```python
from build123d import *

# Parameters (mm, degrees)
BOX006_W     = 90
BOX006_H     = 90
BOX006_DEPTH = 10
FILLET008_R  = 5
BOX007_W     = 100
BOX007_H     = 100
BOX007_DEPTH = 10
FILLET007_R  = 7
BOX008_W     = 94
BOX008_H     = 94
BOX008_DEPTH = 2
FILLET006_R  = 7


with BuildPart() as fillet008:
    # Box006 → Box006 (new body)
    with BuildSketch(Plane(origin=(5, 5, 3), x_dir=(1, 0, 0), z_dir=(0, 0, 1))):
        with Locations((45, 45)):
            Rectangle(BOX006_W, BOX006_H)
    extrude(amount=BOX006_DEPTH)

    # Fillet008
    fillet008_edges = [fillet008.edges().sort_by_distance(p)[0] for p in [
        (5, 5, 8),
        (5, 95, 8),
        (95, 5, 8),
        (95, 95, 8),
    ]]
    fillet(fillet008_edges, radius=FILLET008_R)


with BuildPart() as body_with_fillets003:
    # Box007 → Box007 (new body)
    with BuildSketch(Plane.XY):
        with Locations((50, 50)):
            Rectangle(BOX007_W, BOX007_H)
    extrude(amount=BOX007_DEPTH)

    # Fillet007
    fillet007_edges = [body_with_fillets003.edges().sort_by_distance(p)[0] for p in [
        (0, 0, 5),
        (0, 100, 5),
        (100, 0, 5),
        (100, 100, 5),
    ]]
    fillet(fillet007_edges, radius=FILLET007_R)


with BuildPart() as wet_palette:
    # Box008 → Box008 (new body)
    with BuildSketch(Plane(origin=(3, 3, 10), x_dir=(1, 0, 0), z_dir=(0, 0, 1))):
        with Locations((47, 47)):
            Rectangle(BOX008_W, BOX008_H)
    extrude(amount=BOX008_DEPTH)

    # Fillet006
    fillet006_edges = [wet_palette.edges().sort_by_distance(p)[0] for p in [
        (3, 3, 11),
        (3, 97, 11),
        (97, 3, 11),
        (97, 97, 11),
    ]]
    fillet(fillet006_edges, radius=FILLET006_R)

    # Fusion003: union Body with fillets003
    add(body_with_fillets003.part)

    # Cut002: cut Fillet008
    add(fillet008.part, mode=Mode.SUBTRACT)


with BuildPart() as wet_palette_1:
    # Cut002 placement: moved
    add(wet_palette.part.moved(Location((-110, 0, 0))))


solid = wet_palette_1.part
```
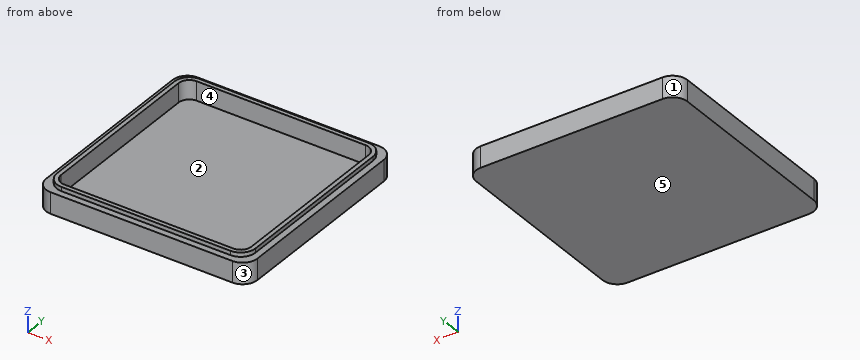
Check sheet for the modelled part. Datum: model origin and axes. Units: mm. Face numbers are marked on the shaded views. A direction names the side the tool comes from. Give positions to 0.01 mm unless a question says otherwise; leave off trailing zeros. Loops run counter-clockwise (first coordinate to the right, second up) from the corner with the lowest first, then second, coordinate; pieces in that order, holes last. Notation, with made-up numbers: M -20,-10.5 L 37,-10.5 A33 ccw 37,25.5 Z; hole C 57.25,50.25 d2. An arc over 180 degrees is marked long. Answer as CSV lines item,"result".
Item 1: Scan lines: L1, parallel to X at y = 47.5, z = 4.25; L2, parallel to Y at x = -94.5, z = 11; L3, parallel to Y at x = -92.5, z = 7.75. Record each from-to range of solid material in increasing order.
Reply:
L1,"-110 to -105, -15 to -10"
L2,"3 to 5, 95 to 97"
L3,"0 to 5, 95 to 100"
Item 2: Sectioned sample at B-B, the plane x = -48. Enter the section's corners in (y, z), then the cut area to 3 significant figures.
Reply:
outline,"M 0,0 L 100,0 L 100,10 L 97,10 L 97,12 L 95,12 L 95,3 L 5,3 L 5,12 L 3,12 L 3,10 L 0,10 Z"
area,"378 mm^2"
Item 3: Sectioned sample at A-A, the plane z = 7.75. Enter the section's corners in (x, y).
Reply:
outline,"M -110,7 A7 ccw -103,0 L -17,0 A7 ccw -10,7 L -10,93 A7 ccw -17,100 L -103,100 A7 ccw -110,93 Z; hole M -105,10 A5 ccw -100,5 L -20,5 A5 ccw -15,10 L -15,90 A5 ccw -20,95 L -100,95 A5 ccw -105,90 Z"
Item 4: Draft check along X on the marked faces 1, 2 and 3. Enter one of: pulls with the +X half, pulls with the -X half, needs draft (parallel to the pull), parting line crosses it, or undercut.
Reply:
face 1,"pulls with the -X half"
face 2,"undercut"
face 3,"pulls with the +X half"
Item 5: Set-up check for the marked faces 4 and 5: record each of +Z, -Z, +X, -X, +Y, -Y from which the full face is reachable in a straight line by a thin tool's end or side.
Reply:
face 4,"+Z"
face 5,"-Z, +X, -X, +Y, -Y"
Item 6: Depth check by flat-ended pin: pin 1 Ø0.6 at (x, z) = (-49, 11.5) entering from +Y; pin 2 Ø1 at (y, z) = (38.5, 11) entering from +X; pin 3 Ø0.6 at (x, z) = (-49, 11) entering from -Y. Enter the tip coordinate at first touch or a pass-through.
Reply:
pin 1,"y = 97"
pin 2,"x = -13"
pin 3,"y = 3"
Item 7: Sectioned sample at C-C, the plane y = 31. Enter the section's corners in (x, z).
Reply:
outline,"M -110,0 L -10,0 L -10,10 L -13,10 L -13,12 L -15,12 L -15,3 L -105,3 L -105,12 L -107,12 L -107,10 L -110,10 Z"
